Design review of the part shown in the three views and the two pictorial views. Dimensions are in mm from the part's minimum x, y and z. Round coordinates to 2 decimals unless told otherwise and drop trailing zeros. Order: outer loops, then holes, each group sorted by start corner. A loop starts at its lowest first (then second) coordinate and runs counter-clockwise, first axis right, second up. Notation, with made-up numbers: M 71,73.25 L 100,73.25 A23 ccw 100,81.25 Z; hole C 59,64.5 d2. An arc over 180 degrees is marked long. Use a Markdown table: item, result. Add a question column.
(1) Take a section at D-D (x = 98). Write out the cut boundary in (y, z), then the cut area to 3 significant figures.
(2) The part is to be moulded in two halves that separate along Y. For the marked faces 1, 2 and 3, say which applies: released by +Y, released by -Y, zero draft, split by the parting line, or undercut.
(3) To check wall thickness, follow probe 1 along Z at (x, y) = (124, 2.05) (3 decimals); probe 2 along X at (y, z) = (4.5, 4.25); probe 3 along Y at (x, z) = (66, 7). State the ranges of each line that lie inside material, in increasing order. Write a range as from..to.
(4) Take a section at B-B (z = 7). Write out the cut boundary in (x, y), then the cut area to 3 significant figures.
(5) Take a section at A-A (x = 124). Write out the cut boundary in (y, z) (3 decimals).
(6) Take a section at C-C (y = 3.75). Count the separate pieces of the cut face and the enclosed holes in it, then the cut area to 3 significant figures.
(7) For pin 1 (6.5 mm diameter, centred on x = 38.5, y = 14.5, fed in from +Z); pin 2 (3 mm diameter, centred on x = 6, z = 4.125, fed in from +Y); pin 3 (1.4 mm diameter, centred on x = 92, y = 20, fed in from -Z); pin 4 (0.8 mm diameter, centred on x = 55.5, y = 19, fed in from +Z), all flat-tipped, find the tip position at first contact; note any pin that passes through.
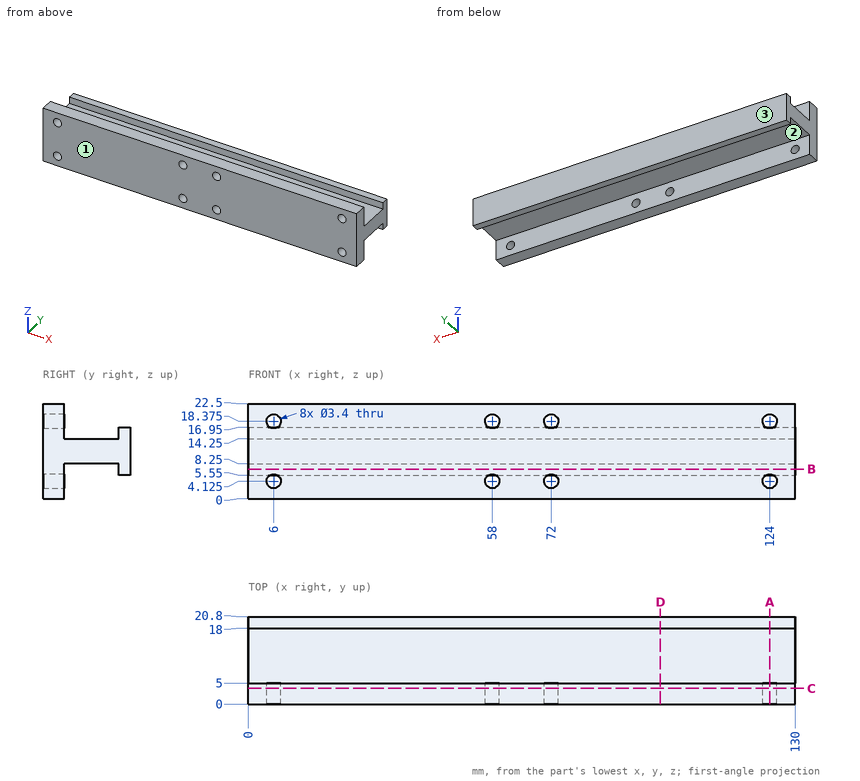
Verdict:
| question | item | result |
|---|---|---|
| 1 | outline | M 0,0 L 5,0 L 5,8.25 L 18,8.25 L 18,5.55 L 20.8,5.55 L 20.8,16.95 L 18,16.95 L 18,14.25 L 5,14.25 L 5,22.5 L 0,22.5 Z |
| 1 | area | 222 mm^2 |
| 2 | face 1 | released by -Y |
| 2 | face 2 | undercut |
| 2 | face 3 | released by +Y |
| 3 | probe 1 | z = 0..2.425, 5.825..16.675, 20.075..22.5 |
| 3 | probe 2 | x = 0..4.3, 7.7..56.3, 59.7..70.3, 73.7..122.3, 125.7..130 |
| 3 | probe 3 | y = 0..5, 18..20.8 |
| 4 | outline | M 0,0 L 130,0 L 130,5 L 0,5 Z; M 0,18 L 130,18 L 130,20.8 L 0,20.8 Z |
| 4 | area | 1,010 mm^2 |
| 5 | outline | M 0,0 L 5,0 L 5,2.425 L 0,2.425 Z; M 0,5.825 L 5,5.825 L 5,8.25 L 18,8.25 L 18,5.55 L 20.8,5.55 L 20.8,16.95 L 18,16.95 L 18,14.25 L 5,14.25 L 5,16.675 L 0,16.675 Z; M 0,20.075 L 5,20.075 L 5,22.5 L 0,22.5 Z |
| 6 | separate pieces | 1 |
| 6 | enclosed holes | 8 |
| 6 | area | 2,850 mm^2 |
| 7 | pin 1 | stops at z = 14.25 |
| 7 | pin 2 | stops at y = 20.8 |
| 7 | pin 3 | stops at z = 5.55 |
| 7 | pin 4 | stops at z = 16.95 |
